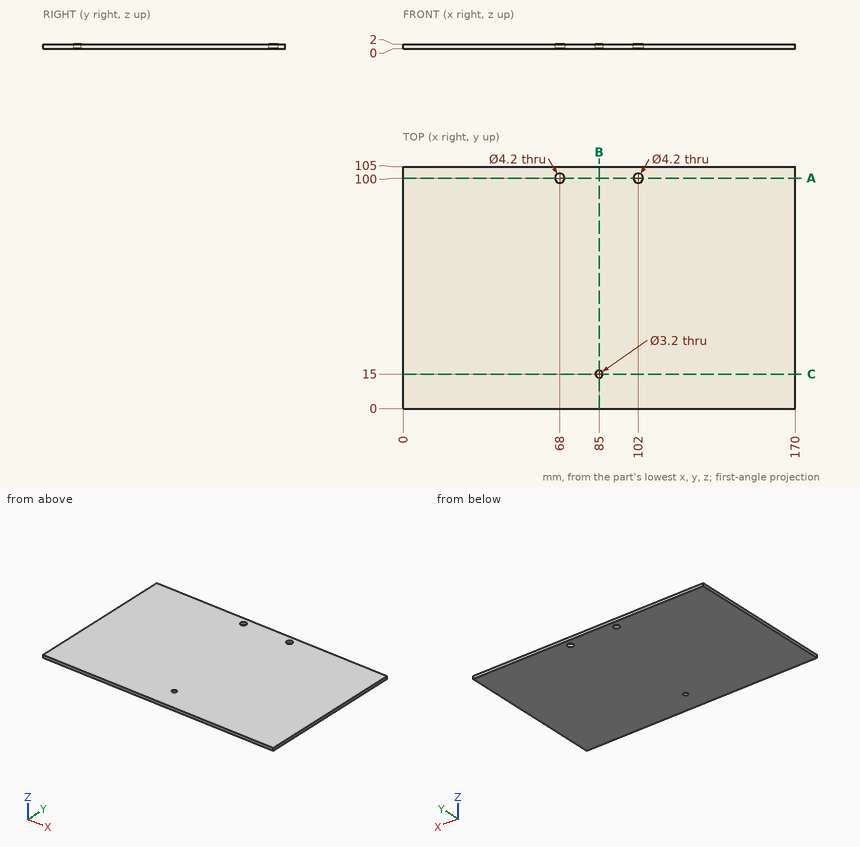
Input: dimensioned drawing with shaded views. Units: mm. Origin: part minimum x, y, z. Give positions to 0.01 mm unless a question says otherwise; leave off trailing zeros. Write each loop counter-clockwise with the first axis right and the second up, starting at its lowest first coordinate (ties: lowest second). Pieces come first, ordered by that corner, then holes.
1. Section query C-C, the plane y = 15. Return loops of the section in (x, z), then the cut area to 3 significant figures.
2. Section query A-A, the plane y = 100. Return loops of the section in (x, z), then the cut area to 3 significant figures.
3. Section query B-B, the plane x = 85. Return loops of the section in (y, z), then the cut area to 3 significant figures.
4. Line query: probe 1 along X at (y, z) = (100, 1.65); probe 2 along Y at (x, z) = (102, 1.2); probe 3 along Y at (x, z) = (85, 1.55). Output: solid intervals per line, ascending.
5. Pin query (flat end, axial travel): P1, Ø5, axis at x = 85, y = 15, coming from the -Z side. Return the tip coordinate at first contact, or that it passes through.
Computed:
1. outline: (0, 0) - (83.4, 0) - (83.4, 2) - (0, 2) - close; (86.6, 0) - (170, 0) - (170, 2) - (86.6, 2) - close
1. area: 334 mm2
2. outline: (0, 0) - (65.9, 0) - (65.9, 2) - (0, 2) - close; (70.1, 0) - (99.9, 0) - (99.9, 2) - (70.1, 2) - close; (104.1, 0) - (170, 0) - (170, 2) - (104.1, 2) - close
2. area: 323 mm2
3. outline: (0, 0) - (13.4, 0) - (13.4, 2) - (0, 2) - close; (16.6, 0) - (105, 0) - (105, 2) - (16.6, 2) - close
3. area: 204 mm2
4. probe 1: x = 0 to 65.9, 70.1 to 99.9, 104.1 to 170
4. probe 2: y = 0 to 97.9, 102.1 to 105
4. probe 3: y = 0 to 13.4, 16.6 to 105
5. P1: stops at z = 0
